Verification items for the finished model (mm, model axes). Face numbers are marked on the shaded views. A direction names the side the tool comes from. Give positions to 0.01 mm unless a question says otherwise; leave off trailing zeros. Loops run counter-clockwise (first coordinate to the right, second up) from the corner with the lowest first, then second, coordinate; pieces in that order, holes last. Notation, with made-up numbers: (77, 9) - (134, 9) arc R26 ccw to (134, 33) - close; hole circle Ø4 at (73, 10.5). An arc over 180 degrees is marked (long way). Use one line per item in the form item = value.
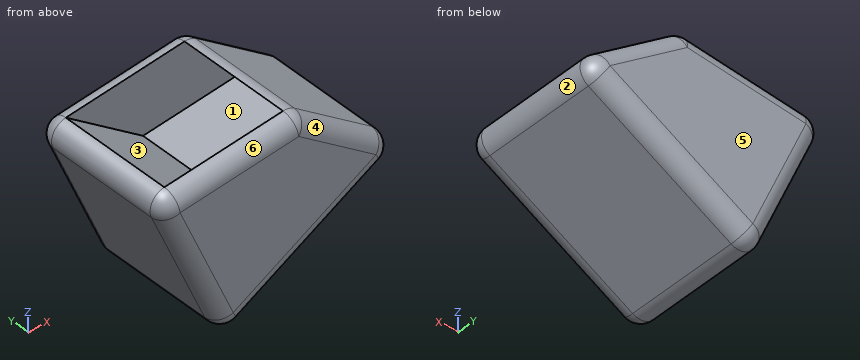
```python
from build123d import *

# Parameters (mm, degrees)
F1_DEPTH   = 46.482
F3_R       = 5.08
F1_FACE1_W = 37.6294337092
F1_FACE1_H = 36.322


# Not quite as in the source:
# - a feature of the source that left no trace in its solid (it failed there, or was rolled back) is left out


with BuildPart() as f1:
    # F0 (on Front) → F1 (new body)
    with BuildSketch(Plane.XZ):
        Polygon((-2.8179630172, 51.4278113842), (-48.9117763937, 45.7918867469), (-27.1732080728, -3.7237356883), (29.5886062086, 28.2802637666), align=None)
    extrude(amount=F1_DEPTH)

    # F3
    f3_edges = [f1.edges().sort_by_distance(p)[0] for p in [
        (-2.817963, -23.241, 51.427811),
        (-48.911776, -23.241, 45.791887),
        (-25.86487, 0, 48.609849),
        (-25.86487, -46.482, 48.609849),
        (-38.042492, 0, 21.034076),
        (1.207699, 0, 12.278264),
        (13.385322, 0, 39.854038),
        (-27.173208, -23.241, -3.723736),
        (29.588606, -23.241, 28.280264),
        (1.207699, -46.482, 12.278264),
        (-38.042492, -46.482, 21.034076),
        (13.385322, -46.482, 39.854038),
    ]]
    fillet(f3_edges, radius=F3_R)

    # F4: sweep along a path in F4_path
    with BuildLine(Plane(origin=(23.0940504855, -41.402, 32.9192317736), x_dir=(0.8137334929, 0, -0.5812381633), z_dir=(-0.5812381633, 0, -0.8137334929))) as f4_path:
        Line((0, 0), (-29.867419561, 0))
    # F1_face1 (on face) → F4 (sweep, cut)
    with BuildSketch(Plane(origin=(-25.8648697054, -23.241, 48.6098490655), x_dir=(1, 0, 0), z_dir=(-0.1213668794, 0, 0.9926077174))):
        with Locations((2.4278813649, 0)):
            Rectangle(F1_FACE1_W, F1_FACE1_H)
    sweep(path=f4_path.line, mode=Mode.SUBTRACT)


solid = f1.part
```
1. Tool access check on the marked faces 1 and 2. Record the directions out of +Z, -Z, +X, -X, +Y, -Y that give a thin tool (end or side, any length) a straight path to the whole face; none if there is none.
Result set:
face_1 = none
face_2 = +X, +Y, -Y
2. Section check A-A, the plane y = -20. Record the cut outline in (x, z).
Result set:
outline = (-46.17, 39.54) - (-29.43, 1.42) arc R5.08 ccw to (-22.28, -0.97) - (22.64, 24.36) arc R5.08 ccw to (23.09, 32.92) - (-1.21, 50.28) arc R5.08 ccw to (-4.78, 51.19) - (19.52, 33.83) - (-17.83, 29.26) - (-42.13, 46.62) arc R5.08 ccw to start
3. Section check B-B, the plane y = -3.5. Record the cut outline in (x, z), then the cut area to 3 significant figures.
Result set:
outline = (-45.93, 39.64) - (-29.2, 1.52) arc R4.83 ccw to (-22.41, -0.75) - (22.51, 24.58) arc R4.83 ccw to (22.95, 32.71) - (-1.36, 50.07) arc R4.83 ccw to (-4.75, 50.94) - (-42.1, 46.37) arc R4.83 ccw to start
area = 2,300 mm²
4. Scan lines: probe 1 along Y at (x, z) = (-14.5, 43.5); probe 2 along Z at (x, y) = (3.5, -36); probe 3 along Z at (x, y) = (14.5, -29). Record each from-to range of solid material in increasing order.
Result set:
probe_1 = -46.48 to -41.4, -5.08 to 0
probe_2 = 13.57 to 31.87, 45.27 to 46.91
probe_3 = 19.77 to 33.21, 37.42 to 39.06
5. Draft check along X on the marked faces 3, 4, 5 and 6. Enter one of: released by +X, released by -X, zero draft, split by the parting line, or undercut.
Result set:
face_3 = undercut
face_4 = released by +X
face_5 = zero draft
face_6 = released by -X
6. Depth check by flat-ended pin: pin 1 Ø4 at (y, z) = (-24, 18.5) entering from +X; pin 2 Ø8 at (y, z) = (-5.5, 13) entering from +X; pin 3 Ø10 at (y, z) = (-6.5, 11.5) entering from -X; pin 4 Ø4 at (x, z) = (-24, 30.5) entering from +Y. Enter the tip coordinate at first touch or a pass-through.
Result set:
pin_1 = 15.79
pin_2 = 9.58
pin_3 = -36.05
pin_4 = 0
7. Section check C-C, the plane y = -43. Record the cut outline in (x, z).
Result set:
outline = (-45.93, 39.64) - (-29.19, 1.52) arc R4.82 ccw to (-22.41, -0.74) - (22.51, 24.59) arc R4.82 ccw to (22.94, 32.71) - (-1.36, 50.07) arc R4.82 ccw to (-4.75, 50.93) - (-42.1, 46.37) arc R4.82 ccw to start
